from build123d import *

# Parameters (mm, degrees)
SKETCH_1_W      = 4.017465015
SKETCH_1_H      = 3.978187255
SKETCH_1_W_2    = 4.077802358
SKETCH_1_H_2    = 4.314220686
SKETCH_1_H_3    = 3.850544283
SKETCH_1_W_3    = 6.026196403
SKETCH_1_H_4    = 4.091203301
EXTRUDE_1_DEPTH = 2


with BuildPart() as part:
    # 草图1 → 凸台-拉伸1 (new body)
    with BuildSketch(Plane.XY):
        with BuildLine():
            Line((-3.013099113, 5.02), (-6.026197287, 5.02))
            Line((-6.026197287, 5.02), (-6.026197287, 3.58112561))
            ThreePointArc((-6.026197287, 3.58112561), (-5.671102411, 2.723845564), (-6.528380473, 3.07894523))
            Line((-6.528380473, 3.07894523), (-9.541479116, 3.07894523))
            ThreePointArc((-9.541479116, 3.07894523), (-10.398757348, 2.723845394), (-10.043662302, 3.58112561))
            Line((-10.043662302, 3.58112561), (-10.043662302, 5.02))
            Line((-10.043662302, 5.02), (-13.056760945, 5.02))
            Line((-13.056760945, 5.02), (-13.056760945, -15.5))
            Line((-13.056760945, -15.5), (-10.043662302, -15.5))
            Line((-10.043662302, -15.5), (-10.043662302, -14.061127012))
            ThreePointArc((-10.043662302, -14.061127012), (-10.398759363, -13.203846763), (-9.541479117, -13.558943832))
            Line((-9.541479117, -13.558943832), (-6.528380473, -13.558943832))
            ThreePointArc((-6.528380473, -13.558943832), (-5.67110042, -13.203846836), (-6.026197287, -14.061126942))
            Line((-6.026197287, -14.061126942), (-6.026197287, -15.5))
            Line((-6.026197287, -15.5), (-3.013099112, -15.5))
            Line((-3.013099112, -15.5), (-3.013099112, -9.541477971))
            Line((-3.013099112, -9.541477971), (3.013099113, -9.541477971))
            Line((3.013099113, -9.541477971), (3.013099113, -15.5))
            Line((3.013099113, -15.5), (6.02619635, -15.5))
            Line((6.02619635, -15.5), (6.02619635, -14.061126942))
            ThreePointArc((6.02619635, -14.061126942), (5.671100318, -13.20384612), (6.528380473, -13.558943762))
            Line((6.528380473, -13.558943762), (9.541479585, -13.558943762))
            ThreePointArc((9.541479585, -13.558943762), (10.398760105, -13.203847022), (10.043661834, -14.061126908))
            Line((10.043661834, -14.061126908), (10.043661834, -15.5))
            Line((10.043661834, -15.5), (13.056760946, -15.5))
            Line((13.056760946, -15.5), (13.056760946, 5.02))
            Line((13.056760946, 5.02), (10.043661833, 5.02))
            Line((10.043661833, 5.02), (10.043661833, 3.58112561))
            ThreePointArc((10.043661833, 3.58112561), (10.398758101, 2.723845772), (9.541479585, 3.07894523))
            Line((9.541479585, 3.07894523), (6.528380474, 3.07894523))
            ThreePointArc((6.528380474, 3.07894523), (5.671102333, 2.723844823), (6.026196353, 3.58112561))
            Line((6.026196353, 3.58112561), (6.026196353, 5.02))
            Line((6.026196353, 5.02), (3.013099113, 5.02))
            Line((3.013099113, 5.02), (3.013099113, -0.938521958))
            Line((3.013099113, -0.938521958), (-3.013099113, -0.938521958))
            Line((-3.013099113, -0.938521958), (-3.013099113, 5.02))
        make_face()
        with Locations((-8.034929795, -8.556751552)):
            Rectangle(SKETCH_1_W, SKETCH_1_H, mode=Mode.SUBTRACT)
        with Locations((8.06509753, -8.724768268)):
            Rectangle(SKETCH_1_W_2, SKETCH_1_H_2, mode=Mode.SUBTRACT)
        with Locations((8.06509753, -1.788857431)):
            Rectangle(SKETCH_1_W_2, SKETCH_1_H_3, mode=Mode.SUBTRACT)
        with Locations((-4.68e-07, -5.278413187)):
            Rectangle(SKETCH_1_W_3, SKETCH_1_H_4, mode=Mode.SUBTRACT)
        with Locations((-8.034929795, -1.788857431)):
            Rectangle(SKETCH_1_W, SKETCH_1_H_3, mode=Mode.SUBTRACT)
    extrude(amount=EXTRUDE_1_DEPTH)


solid = part.part
Check sheet for the modelled part. Datum: model origin and axes. Units: mm. A direction names the side the tool comes from. Give positions to 0.01 mm unless a question says otherwise; leave off trailing zeros. Order: outer loops, then holes, each group sorted by start corner. A loop starts at its lowest first (then second) coordinate and runs counter-clockwise, first axis right, second up. Notation, with made-up numbers: M -23,23.25 L -9,23.25 A17 ccw -9,48.25 Z; hole C 45,-27 d2. An arc over 180 degrees is marked long. Answer as CSV lines item,"result". Start each with the question number.
Item 1: Cross-section at D-D on z = 1.7. State how many separate pieces and enclosed holes the cut face has, plus the area to 3 significant figures.
Item 2: Cross-section at C-C on x = 2. Enter the section's corners in (y, z), plus the area to 3 significant figures.
Item 3: Thickness scan on line 1 (X direction, y = -2, z = 1.6); line 2 (Y direction, x = -8, z = 1.55); line 3 (X direction, y = -7, z = 1.55). Record the ranges inside material, lowest first. Write a range as [from, to].
Item 4: Gauge pin test, flat end, axial feed: P1, Ø0.6, axis at x = 8, z = 0.5, coming from the -Y side. Record the tip position at first contact, or that the pin passes through.
Item 5: Tool access check on faces 1 (the face through (-8, 3.079, 1)), 2 (the face through (12, 5.02, 1)), 3 (the face through (-8, -13.559, 1)), 4 (the face through (0, -3.233, 1)). Record the directions out of +Z, -Z, +X, -X, +Y, -Y that give a thin tool (end or side, any length) a straight path to the whole face; none if there is none.
Item 6: Cross-section at B-B on y = -10.25. Enter the section's corners in (x, z), plus the area to 3 significant figures.
Item 7: Cross-section at A-A on x = -8. Enter the section's corners in (y, z), plus the area to 3 significant figures.
Item 8: Mould release check, pull along Y, two halves, no side actions. Record for faces 5 (the face through (0, -7.324, 1)), 6 (the face through (0, -3, 0)), 7 (the face through (8, 3.079, 1)): +Y half, -Y half, draft (parallel to the pull), parting line (faces both ways), or undercut.
Established:
1,separate pieces,"1"
1,enclosed holes,"5"
1,area,"339 mm^2"
2,outline,"M -9.54,0 L -7.32,0 L -7.32,2 L -9.54,2 Z; M -3.23,0 L -0.94,0 L -0.94,2 L -3.23,2 Z"
2,area,"9.02 mm^2"
3,line 1,"x = [-13.06, -10.04], [-6.03, 6.03], [10.1, 13.06]"
3,line 2,"y = [-13.56, -10.55], [-6.57, -3.71], [0.14, 3.08]"
3,line 3,"x = [-13.06, -10.04], [-6.03, -3.01], [3.01, 6.03], [10.1, 13.06]"
4,P1,"stops at y = -13.56"
5,face 1,"+Z, -Z, +Y"
5,face 2,"+Z, -Z, +X, -X, +Y"
5,face 3,"+Z, -Z, -Y"
5,face 4,"+Z, -Z"
6,outline,"M -13.06,0 L -10.04,0 L -10.04,2 L -13.06,2 Z; M -6.03,0 L -3.01,0 L -3.01,2 L -6.03,2 Z; M 3.01,0 L 6.03,0 L 6.03,2 L 3.01,2 Z; M 10.1,0 L 13.06,0 L 13.06,2 L 10.1,2 Z"
6,area,"24.0 mm^2"
7,outline,"M -13.56,0 L -10.55,0 L -10.55,2 L -13.56,2 Z; M -6.57,0 L -3.71,0 L -3.71,2 L -6.57,2 Z; M 0.14,0 L 3.08,0 L 3.08,2 L 0.14,2 Z"
7,area,"17.6 mm^2"
8,face 5,"undercut"
8,face 6,"draft"
8,face 7,"+Y half"
